from build123d import *

# Parameters (mm, degrees)
F0_W     = 45
F0_H     = 2060
F0_W_2   = 22.5
F1_DEPTH = 50
F0_W_3   = 499.5
F2_DEPTH = 12
F0_W_4   = 531
F3_DEPTH = 25


# Not quite as in the source:
# - a feature names something its author has since deleted; it is built from what else it names


with BuildPart() as f1:
    # F0 (on Front) → F1 (new body)
    with BuildSketch(Plane.XZ):
        with Locations((832.5, 0)):
            Rectangle(F0_W, F0_H)
        Polygon((288, -1075), (855, -1075), (855, -1030), (810, -1030), (310.5, -1030), (288, -1030), align=None)
        Polygon((-855, -1075), (288, -1075), (288, -1030), (265.5, -1030), (-265.5, -1030), (-310.5, -1030), (-810, -1030), (-855, -1030), align=None)
        with Locations((-832.5, 0)):
            Rectangle(F0_W, F0_H)
        with Locations((276.75, 0)):
            Rectangle(F0_W_2, F0_H)
        Polygon((810, 1030), (855, 1030), (855, 1075), (288, 1075), (288, 1030), (310.5, 1030), align=None)
        Polygon((265.5, 1030), (288, 1030), (288, 1075), (-855, 1075), (-855, 1030), (-810, 1030), (-310.5, 1030), (-265.5, 1030), align=None)
        with Locations((-288, 0)):
            Rectangle(F0_W, F0_H)
        with Locations((299.25, 0)):
            Rectangle(F0_W_2, F0_H)
    extrude(amount=-F1_DEPTH)

    # F0 (on Front) → F2 (join)
    with BuildSketch(Plane.XZ):
        Polygon((855, -1030), (855, -1075), (288, -1075), (288, -1125), (912, -1125), (912, 1175), (288, 1175), (288, 1075), (855, 1075), (855, 1030), align=None)
        with Locations((560.25, 0)):
            Rectangle(F0_W_3, F0_H)
        Polygon((288, -1075), (855, -1075), (855, -1030), (810, -1030), (310.5, -1030), (288, -1030), align=None)
        with Locations((832.5, 0)):
            Rectangle(F0_W, F0_H)
        Polygon((810, 1030), (855, 1030), (855, 1075), (288, 1075), (288, 1030), (310.5, 1030), align=None)
        with Locations((299.25, 0)):
            Rectangle(F0_W_2, F0_H)
    extrude(amount=F2_DEPTH)

    # F0 (on Front) → F3 (join)
    with BuildSketch(Plane.XZ):
        Polygon((288, -1125), (288, -1075), (-855, -1075), (-855, -1030), (-855, 1030), (-855, 1075), (288, 1075), (288, 1175), (-912, 1175), (-912, -1125), align=None)
        with Locations((-288, 0)):
            Rectangle(F0_W, F0_H)
        Polygon((265.5, 1030), (288, 1030), (288, 1075), (-855, 1075), (-855, 1030), (-810, 1030), (-310.5, 1030), (-265.5, 1030), align=None)
        with Locations((-832.5, 0)):
            Rectangle(F0_W, F0_H)
        with Locations((-560.25, 0)):
            Rectangle(F0_W_3, F0_H)
        Rectangle(F0_W_4, F0_H)
        Polygon((-855, -1075), (288, -1075), (288, -1030), (265.5, -1030), (-265.5, -1030), (-310.5, -1030), (-810, -1030), (-855, -1030), align=None)
        with Locations((276.75, 0)):
            Rectangle(F0_W_2, F0_H)
    extrude(amount=F3_DEPTH)


solid = f1.part
Input: part model. Units: mm. Frame: model coordinates. A direction names the side the tool comes from. Give positions to 0.01 mm unless a question says otherwise; leave off trailing zeros. Loops run counter-clockwise (first coordinate to the right, second up) from the corner with the lowest first, then second, coordinate; pieces in that order, holes last. Notation, with made-up numbers: M 37.5,-3 L 46.5,-3 A13 cw 46.5,10 Z; hole C 15.5,28.5 d5. An arc over 180 degrees is marked long. Use one line per item in the form item = value.
1. First-contact query: pin 1 (5 mm diameter, centred on y = 31.5, z = -228.5, fed in from -X); pin 2 (6.5 mm diameter, centred on y = -20.5, z = -490.5, fed in from +X); pin 3 (1 mm diameter, centred on x = 664, y = 26, fed in from -Z). Flat tips, straight axial feed; report the tip coordinate or a pass-through.
Numbers:
pin_1 = -855
pin_2 = 288
pin_3 = -1075
2. Line query: L1, parallel to X at y = 20, z = -252.5; L2, parallel to Z at x = -645.5, y = 44.5; L3, parallel to Y at x = 428, z = 779.5. Output: solid intervals per line, ascending.
Numbers:
L1 = -855 to -810, -310.5 to -265.5, 265.5 to 310.5, 810 to 855
L2 = -1075 to -1030, 1030 to 1075
L3 = -12 to 0
3. Pull-direction query (Z, two-part tool) for faces 4 (the face through (310.5, 25, -14)), 5 (the face through (-320, -25, 41)), 6 (the face through (12, 25, 1075)); classes: released by +Z, released by -Z, zero draft, split by the parting line, or undercut.
Numbers:
face_4 = undercut
face_5 = zero draft
face_6 = released by +Z
4. Reachability of faces 1 (the face through (855, 25, -15)), 2 (the face through (-827, 50, 5)), 3 (the face through (-265.5, 25, -14)) from +Z, -Z, +X, -X, +Y, -Y: full face, straight path, thin tool, end or side. Return the list, or none.
Numbers:
face_1 = +Z, -Z, +X, +Y
face_2 = +Z, -Z, +X, -X, +Y
face_3 = +Y
5. Section query A-A, the plane y = 26.5. Return the cut outline in (x, z).
Numbers:
outline = M -855,-1075 L 855,-1075 L 855,1075 L -855,1075 Z; hole M -810,-1030 L -310.5,-1030 L -310.5,1030 L -810,1030 Z; hole M -265.5,-1030 L 265.5,-1030 L 265.5,1030 L -265.5,1030 Z; hole M 310.5,-1030 L 810,-1030 L 810,1030 L 310.5,1030 Z
6. Section query B-B, the plane z = 836. Return the cut outline in (x, y).
Numbers:
outline = M -912,-25 L 288,-25 L 288,-12 L 912,-12 L 912,0 L 855,0 L 855,50 L 810,50 L 810,0 L 310.5,0 L 310.5,50 L 265.5,50 L 265.5,0 L -265.5,0 L -265.5,50 L -310.5,50 L -310.5,0 L -810,0 L -810,50 L -855,50 L -855,0 L -912,0 Z
7. Section query C-C, the plane x = 402. Return the cut outline in (y, z), and give its area (3 significant figures).
Numbers:
outline = M -12,-1125 L 0,-1125 L 0,-1075 L 50,-1075 L 50,-1030 L 0,-1030 L 0,1030 L 50,1030 L 50,1075 L 0,1075 L 0,1175 L -12,1175 Z
area = 32,100 mm²
8. Section query D-D, the plane x = -770.5. Return the cut outline in (y, z).
Numbers:
outline = M -25,-1125 L 0,-1125 L 0,-1075 L 50,-1075 L 50,-1030 L 0,-1030 L 0,1030 L 50,1030 L 50,1075 L 0,1075 L 0,1175 L -25,1175 Z
